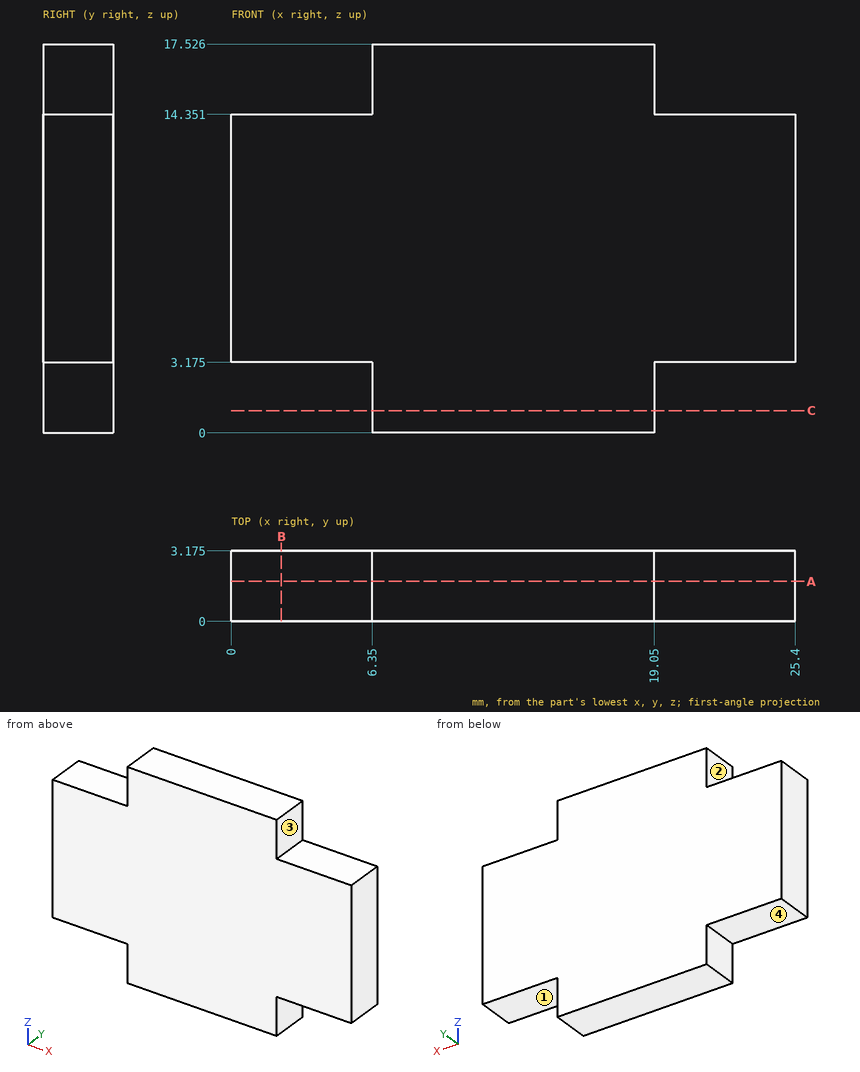
Input: dimensioned drawing with shaded views. Units: mm. Origin: part minimum x, y, z. A direction names the side the tool comes from. Coordinates: 2 decimals unless noted, no trailing zeros. Order: outer loops, then holes, each group sorted by start corner. A loop starts at its lowest first (then second) coordinate and runs counter-clockwise, first axis right, second up.
(1) Access query for the marked faces 1, 2, 3 and 4. Directions: +Z, -Z, +X, -X, +Y, -Y. A direction counts if a zero-diameter tool reaches every point of the face in a straight line with its end or side. Return the directions, or none.
(2) Section query C-C (z = 1). Return the cut outline in (x, y) (3 decimals), plus the area to 3 significant figures.
(3) Section query B-B (x = 2.25). Return the cut outline in (y, z) (3 decimals), plus the area to 3 significant figures.
(4) First-contact query: pin 1 (1.6 mm diameter, centred on y = 1, z = 16, fed in from -X); pin 2 (1 mm diameter, centred on y = 1.5, z = 15.5, fed in from +X); pin 3 (1 mm diameter, centred on x = 18.5, z = 12, fed in from -Y); pin 4 (1.6 mm diameter, centred on x = 23.5, y = 2, fed in from -Z) (3 decimals). Flat tips, straight axial feed; report the tip coordinate or a pass-through.
(5) Material intervals for probe 1 along Z at (x, y) = (20.25, 1.55) (3 decimals); probe 2 along X at (y, z) = (0.35, 2), sorted ascending.
(6) Section query A-A (y = 1.8). Return the cut outline in (x, z) (3 decimals).
Solution:
1. face 1: -Z, +X, +Y, -Y
1. face 2: +Z, -X, +Y, -Y
1. face 3: +Z, +X, +Y, -Y
1. face 4: -Z, -X, +Y, -Y
2. outline: (6.35, 0) - (19.05, 0) - (19.05, 3.175) - (6.35, 3.175) - close
2. area: 40.3 mm2
3. outline: (0, 3.175) - (3.175, 3.175) - (3.175, 14.351) - (0, 14.351) - close
3. area: 35.5 mm2
4. pin 1: stops at x = 6.35
4. pin 2: stops at x = 19.05
4. pin 3: stops at y = 0
4. pin 4: stops at z = 3.175
5. probe 1: z = 3.175 to 14.351
5. probe 2: x = 6.35 to 19.05
6. outline: (0, 3.175) - (6.35, 3.175) - (6.35, 0) - (19.05, 0) - (19.05, 3.175) - (25.4, 3.175) - (25.4, 14.351) - (19.05, 14.351) - (19.05, 17.526) - (6.35, 17.526) - (6.35, 14.351) - (0, 14.351) - close
